```python
from build123d import *

# Parameters (mm, degrees)
SKETCH1_W           = 203.2
SKETCH1_H           = 203.2
SKETCH1_W_2         = 190.5
SKETCH1_H_2         = 190.5
BOSS_EXTRUDE1_DEPTH = 90.678
SKETCH2_W           = 203.2
SKETCH2_H           = 203.2
BOSS_EXTRUDE2_DEPTH = 12.7
SKETCH4_R           = 38.1
CUT_EXTRUDE3_DEPTH  = 178.008844084


with BuildPart() as part:
    # Sketch1 → Boss-Extrude1 (new body)
    with BuildSketch(Plane(origin=(0, 0, 0), x_dir=(1, 0, 0), z_dir=(0, 1, 0))):
        Rectangle(SKETCH1_W, SKETCH1_H)
        Rectangle(SKETCH1_W_2, SKETCH1_H_2, mode=Mode.SUBTRACT)
    extrude(amount=BOSS_EXTRUDE1_DEPTH)

    # Sketch2 → Boss-Extrude2 (add)
    with BuildSketch(Plane(origin=(0, 90.678, 0), x_dir=(1, 0, 0), z_dir=(0, 1, 0))):
        Rectangle(SKETCH2_W, SKETCH2_H)
    extrude(amount=BOSS_EXTRUDE2_DEPTH)

    # Sketch4 → Cut-Extrude3 (cut, through all)
    with BuildSketch(Plane(origin=(0, 103.378, 0), x_dir=(1, 0, 0), z_dir=(0, 1, 0))):
        with Locations(Location((0, 0, 0), (0, 0, 270))):
            Circle(SKETCH4_R)
    extrude(amount=-CUT_EXTRUDE3_DEPTH, mode=Mode.SUBTRACT)


solid = part.part
```
Here's how the part is built. I have some questions about the finished solid (model axes, mm). A direction names the side the tool comes from. Give positions to 0.01 mm unless a question says otherwise; leave off trailing zeros. Loops run counter-clockwise (first coordinate to the right, second up) from the corner with the lowest first, then second, coordinate; pieces in that order, holes last. Notation, with made-up numbers: M 53.25,17.5 L 81.25,17.5 A6 cw 81.25,21.5 Z; hole C 29,72 d5. An arc over 180 degrees is marked long. Put each result on its own line as item: value. Start each with the question number.
(1) Will this pin go through, and if not, where does the flat tip stop? pin 1 Ø1.5 at (x, z) = (-48, -50) entering from -Y.
(2) For faces 1 (the flat face through (-8, 0, 97)), 2 (the flat face through (95.25, 45, 1)), which set-ups out of +Z, -Z, +X, -X, +Y, -Y let a thin tool reach every point of the face, with its end or its side?
(3) I want a section at D-D on x = -60.5. Please give me the cut outline in (y, z), then the cut area to 3 significant figures.
(4) I want a section at B-B on z = 0. Please give me the cut outline in (x, y).
(5) I need wall thicknesses on line 1 along X through (y, z) = (7, 76); line 2 along X through (y, z) = (97.25, 0). Which ranges of each line are inside material? Lowest first, please. Write a range as [from, to].
(6) I want a section at A-A on x = 0. Please give me the cut outline in (y, z).
(7) I want a section at C-C on y = 65. Please give me the cut outline in (x, z), then the cut area to 3 significant figures.
(8) If we mould it in two halves opening along X, with no side actions, what happens to faces 3 (the flat face through (-1, 51, 101.6)), 4 (the flat face through (-101.6, 51, 1)), 5 (the flat face through (-1, 45, -95.25))? For each: +X half, -X half, draft (parallel to the pull), parting line (faces both ways), or undercut.
Answer block:
1. pin 1: y = 90.68
2. face 1: +Z, -Z, +X, -X, -Y
2. face 2: -Y
3. outline: M 0,-101.6 L 103.38,-101.6 L 103.38,101.6 L 0,101.6 L 0,95.25 L 90.68,95.25 L 90.68,-95.25 L 0,-95.25 Z
3. area: 3,730 mm^2
4. outline: M -101.6,0 L -95.25,0 L -95.25,90.68 L -38.1,90.68 L -38.1,103.38 L -101.6,103.38 Z; M 38.1,90.68 L 95.25,90.68 L 95.25,0 L 101.6,0 L 101.6,103.38 L 38.1,103.38 Z
5. line 1: [-101.6, -95.25], [95.25, 101.6]
5. line 2: [-101.6, -38.1], [38.1, 101.6]
6. outline: M 0,-101.6 L 103.38,-101.6 L 103.38,-38.1 L 90.68,-38.1 L 90.68,-95.25 L 0,-95.25 Z; M 0,95.25 L 90.68,95.25 L 90.68,38.1 L 103.38,38.1 L 103.38,101.6 L 0,101.6 Z
7. outline: M -101.6,-101.6 L 101.6,-101.6 L 101.6,101.6 L -101.6,101.6 Z; hole M -95.25,-95.25 L 95.25,-95.25 L 95.25,95.25 L -95.25,95.25 Z
7. area: 5,000 mm^2
8. face 3: draft
8. face 4: -X half
8. face 5: undercut
